```python
from build123d import *

# Parameters (mm, degrees)
F0_R     = 1.5
F1_DEPTH = 0.5


with BuildPart() as f1:
    # F0 (on Front) → F1 (new body)
    with BuildSketch(Plane.XZ):
        with BuildLine():
            Line((38, 40), (2, 40))
            ThreePointArc((2, 40), (0.585786, 39.414214), (0, 38))
            Line((0, 38), (0, 11))
            Line((0, 11), (40, 11))
            Line((40, 11), (40, 38))
            ThreePointArc((40, 38), (39.414214, 39.414214), (38, 40))
        make_face()
        with Locations((10, 14)):
            Circle(F0_R, mode=Mode.SUBTRACT)
        with Locations((30, 14)):
            Circle(F0_R, mode=Mode.SUBTRACT)
    extrude(amount=F1_DEPTH)


solid = f1.part
```
Check sheet for the modelled part. Datum: model origin and axes. Units: mm. Round coordinates to 2 decimals unless told otherwise and drop trailing zeros. Write each loop counter-clockwise with the first axis right and the second up, starting at its lowest first coordinate (ties: lowest second). Pieces come first, ordered by that corner, then holes. Notation, with made-up numbers: M -30.5,-36 L 6.5,-36 A20 ccw 6.5,-24 Z; hole C 2.25,-17 d9. An arc over 180 degrees is marked long. Write item = value, one per line. Start each with the question number.
1. Section check C-C, the plane x = 10.5. Record the cut outline in (y, z).
2. Release check for a two-part mould opening along Z. For faces 1 (the flat face through (20, 0, 26)), 2 (the cylindrical face through (28.5, -0.25, 14.07)), 3 (the cylindrical face through (0.6, -0.25, 39.43)) record: pulls with the +Z half, pulls with the -Z half, needs draft (parallel to the pull), parting line crosses it, or undercut.
3. Section check B-B, the plane z = 14. Record the cut outline in (x, y), then the cut area to 3 significant figures.
4. Scan lines: line 1 (Z direction, x = 30, y = -0.05); line 2 (X direction, y = -0.35, z = 15); line 3 (Z direction, x = 29.5, y = -0.2). Record each from-to range of solid material in increasing order. Write a range as [from, to].
5. Section check A-A, the plane x = 30. Record the cut outline in (y, z).
Results found:
q1.outline = M -0.5,11 L 0,11 L 0,12.59 L -0.5,12.59 Z; M -0.5,15.41 L 0,15.41 L 0,40 L -0.5,40 Z
q2.face_1 = needs draft
q2.face_2 = undercut
q2.face_3 = pulls with the +Z half
q3.outline = M 0,-0.5 L 8.5,-0.5 L 8.5,0 L 0,0 Z; M 11.5,-0.5 L 28.5,-0.5 L 28.5,0 L 11.5,0 Z; M 31.5,-0.5 L 40,-0.5 L 40,0 L 31.5,0 Z
q3.area = 17.0 mm^2
q4.line_1 = [11, 12.5], [15.5, 40]
q4.line_2 = [0, 8.88], [11.12, 28.88], [31.12, 40]
q4.line_3 = [11, 12.59], [15.41, 40]
q5.outline = M -0.5,11 L 0,11 L 0,12.5 L -0.5,12.5 Z; M -0.5,15.5 L 0,15.5 L 0,40 L -0.5,40 Z
